```python
from build123d import *

# Parameters (mm, degrees)
BOSS_EXTRUDE1_DEPTH      = 14.5
BOSS_EXTRUDE1_DEPTH_BACK = 18
SKETCH1_W                = 13.75
SKETCH1_H                = 13.75
CUT_EXTRUDE1_DEPTH       = 21.458036318
CUT_EXTRUDE1_DEPTH_BACK  = 21.458036318
SKETCH2_R                = 1.4
FILLET1_R                = 1
FILLET2_R                = 1
SKETCH3_R                = 1.4
CUT_EXTRUDE2_DEPTH       = 34.923166863


with BuildPart() as part:
    # Sketch1 → Boss-Extrude1 (new, two sides: drawn at the far end of the back side and taken through both)
    with BuildSketch(Plane.XY.offset(-BOSS_EXTRUDE1_DEPTH_BACK)):
        Rectangle(SKETCH1_W, SKETCH1_H)
    extrude(amount=BOSS_EXTRUDE1_DEPTH + BOSS_EXTRUDE1_DEPTH_BACK)

    # Sketch2 → Cut-Extrude1 (cut, two sides: drawn at the far end of the back side and taken through both)
    with BuildSketch(Plane(origin=(0, 0, 0), x_dir=(1, 0, 0), z_dir=(0, 1, 0)).offset(-CUT_EXTRUDE1_DEPTH_BACK)):
        with Locations(Location((0, 0, 0), (0, 0, 270))):
            Circle(SKETCH2_R)
        with Locations(Location((0, 13.5, 0), (0, 0, 270))):
            Circle(SKETCH2_R)
    extrude(amount=CUT_EXTRUDE1_DEPTH + CUT_EXTRUDE1_DEPTH_BACK, mode=Mode.SUBTRACT)

    # Fillet1
    fillet1_edges = [part.edges().sort_by_distance(p)[0] for p in [
        (6.875, 0, 14.5),
        (-6.875, 0, -18),
        (0, 6.875, 14.5),
        (-6.875, 0, 14.5),
        (0, -6.875, 14.5),
        (0, -6.875, -18),
        (6.875, 0, -18),
        (6.875, -6.875, -1.75),
        (-6.875, -6.875, -1.75),
        (-6.875, 6.875, -1.75),
        (6.875, 6.875, -1.75),
        (0, 6.875, -18),
    ]]
    fillet(fillet1_edges, radius=FILLET1_R)

    # Fillet2
    fillet2_edges = [part.edges().sort_by_distance(p)[0] for p in [
        (0, -6.875, -1.4),
        (0, 6.875, -1.4),
        (0, -6.875, -14.9),
        (0, 6.875, -14.9),
    ]]
    fillet(fillet2_edges, radius=FILLET2_R)

    # Sketch3 → Cut-Extrude2 (cut, through all)
    with BuildSketch(Plane.XY.offset(14.5)):
        with Locations((-3.5, 0)):
            Circle(SKETCH3_R)
        with Locations((3.5, 0)):
            Circle(SKETCH3_R)
    extrude(amount=-CUT_EXTRUDE2_DEPTH, mode=Mode.SUBTRACT)


solid = part.part
```
Model file for the job. Use its own axes, mm. Coordinates: 2 decimals unless noted, no trailing zeros. Loops run counter-clockwise (first coordinate to the right, second up) from the corner with the lowest first, then second, coordinate; pieces in that order, holes last. Notation, with made-up numbers: (70, -14.75) - (84, -14.75) arc R38 cw to (84, 23.25) - close; hole circle Ø2 at (-13, -35). An arc over 180 degrees is marked (long way). Write item = value, one per line. Start each with the question number.
Item 1: Saw through at B-B, the plane y = 0. List the corners of the cut face in (x, z) (3 decimals).
Item 2: Drop a flat-ended pin along its axis: pin 1 Ø2.5 at (x, y) = (-3.5, 0) entering from +Z. Give the stop position or say it passes through.
Item 3: Wall check: probe 1 along Z at (x, y) = (0, -0.25); probe 2 along Z at (x, y) = (-0.75, 3.5); probe 3 along Z at (x, y) = (6, 2.75). Give the ranges that are in metal, low to high. Write a range as [from, to].
Item 4: Saw through at A-A, the plane z = -13.5. List the corners of the cut face in (x, y) (3 decimals), then the cut area to 3 significant figures.
Item 5: Saw through at C-C, the plane x = 0. List the corners of the cut face in (y, z) (3 decimals).
Item 6: Saw through at D-D, the plane y = -5. List the corners of the cut face in (x, z) (3 decimals), then the cut area to 3 significant figures.
Item 7: Pull direction X, two halves, no side cores. Call faces 1 (the face through (-2.21, -0.54, -1.52)), 2 (the face through (0.08, 6.59, 14.2)), 3 (the face through (6.574, 0.082, 14.215)): +X half, -X half, draft (parallel to the pull), parting line (faces both ways), or undercut.
Answers:
q1.outline = (-6.875, -17) arc R1 ccw to (-5.875, -18) - (-4.9, -18) - (-4.9, 14.5) - (-5.875, 14.5) arc R1 ccw to (-6.875, 13.5) - close; (-2.1, -18) - (2.1, -18) - (2.1, 14.5) - (-2.1, 14.5) - close; (4.9, -18) - (5.875, -18) arc R1 ccw to (6.875, -17) - (6.875, 13.5) arc R1 ccw to (5.875, 14.5) - (4.9, 14.5) - close; hole circle Ø2.8 at (0, -13.5); hole circle Ø2.8 at (0, 0)
q2.pin_1 = through
q3.probe_1 = [-18, -14.9], [-12.1, -1.4], [1.4, 14.5]
q3.probe_2 = [-18, -14.68], [-12.32, -1.18], [1.18, 14.5]
q3.probe_3 = [-17.99, 14.49]
q4.outline = (-6.875, -5.875) arc R1 ccw to (-5.875, -6.875) - (-2.4, -6.875) arc R1 ccw to (-1.4, -5.875) - (-1.4, 5.875) arc R1 ccw to (-2.4, 6.875) - (-5.875, 6.875) arc R1 ccw to (-6.875, 5.875) - close; (1.4, -5.875) arc R1 ccw to (2.4, -6.875) - (5.875, -6.875) arc R1 ccw to (6.875, -5.875) - (6.875, 5.875) arc R1 ccw to (5.875, 6.875) - (2.4, 6.875) arc R1 ccw to (1.4, 5.875) - close; hole circle Ø2.8 at (-3.5, 0); hole circle Ø2.8 at (3.5, 0)
q4.area = 137 mm2
q5.outline = (-6.875, -17) arc R1 ccw to (-5.875, -18) - (5.875, -18) arc R1 ccw to (6.875, -17) - (6.875, -15.9) arc R1 ccw to (5.875, -14.9) - (-5.875, -14.9) arc R1 ccw to (-6.875, -15.9) - close; (-6.875, -11.1) arc R1 ccw to (-5.875, -12.1) - (5.875, -12.1) arc R1 ccw to (6.875, -11.1) - (6.875, -2.4) arc R1 ccw to (5.875, -1.4) - (-5.875, -1.4) arc R1 ccw to (-6.875, -2.4) - close; (-6.875, 2.4) arc R1 ccw to (-5.875, 1.4) - (5.875, 1.4) arc R1 ccw to (6.875, 2.4) - (6.875, 13.5) arc R1 ccw to (5.875, 14.5) - (-5.875, 14.5) arc R1 ccw to (-6.875, 13.5) - close
q6.outline = (-6.875, -17) arc R1 ccw to (-5.875, -18) - (5.875, -18) arc R1 ccw to (6.875, -17) - (6.875, 13.5) arc R1 ccw to (5.875, 14.5) - (-5.875, 14.5) arc R1 ccw to (-6.875, 13.5) - close; hole circle Ø2.8 at (0, -13.5); hole circle Ø2.8 at (0, 0)
q6.area = 434 mm2
q7.face_1 = undercut
q7.face_2 = draft
q7.face_3 = +X half
